```python
from build123d import *

# Parameters (mm, degrees)
EXTRUDE1_DEPTH                                    = 177.8
F_6_32_TAPPED_HOLE1_D                             = 2.7051
F_6_32_TAPPED_HOLE1_DEPTH                         = 9.38784
F_6_32_TAPPED_HOLE1_CBORE_D                       = 3.5052
F_6_32_TAPPED_HOLE1_CBORE_DEPTH                   = 7.0104
F_6_32_TAPPED_HOLE1_TIP                           = 0.81269403
F_6_32_TAPPED_HOLE2_D                             = 2.7051
F_6_32_TAPPED_HOLE2_DEPTH                         = 9.38784
F_6_32_TAPPED_HOLE2_TIP                           = 0.81269403
F_6_32_TAPPED_HOLE3_D                             = 2.7051
F_6_32_TAPPED_HOLE3_DEPTH                         = 9.38784
F_6_32_TAPPED_HOLE3_TIP                           = 0.81269403
CSK_FOR_6_FLAT_HEAD_MACHINE_SCREW_100_D           = 3.7973
CSK_FOR_6_FLAT_HEAD_MACHINE_SCREW_100_DEPTH       = 12.7
CSK_FOR_6_FLAT_HEAD_MACHINE_SCREW_100_CSINK_D     = 7.0866
CSK_FOR_6_FLAT_HEAD_MACHINE_SCREW_100_CSINK_ANGLE = 100
CSK_FOR_6_FLAT_HEAD_MACHINE_SCREW_100_TIP         = 1.140824014


with BuildPart() as part:
    # Sketch1 → Extrude1 (new body)
    with BuildSketch(Plane(origin=(0, 0, 0), x_dir=(1, 0, 0), z_dir=(0, 1, 0))):
        with BuildLine():
            Line((0, -2.54), (0, -101.092))
            ThreePointArc((0, -101.092), (0.743948776, -102.888051224), (2.54, -103.632))
            Line((2.54, -103.632), (50.8, -103.632))
            Line((50.8, -103.632), (50.8, -100.632))
            Line((50.8, -100.632), (5.54, -100.632))
            ThreePointArc((5.54, -100.632), (3.743948776, -99.888051224), (3, -98.092))
            Line((3, -98.092), (3, -5.54))
            ThreePointArc((3, -5.54), (3.743948776, -3.743948776), (5.54, -3))
            Line((5.54, -3), (50.8, -3))
            Line((50.8, -3), (50.8, 0))
            Line((50.8, 0), (2.54, 0))
            ThreePointArc((2.54, 0), (0.743948776, -0.743948776), (0, -2.54))
        make_face()
    extrude(amount=-EXTRUDE1_DEPTH)

    # #6-32 Tapped Hole1
    with Locations(Plane.ZY):
        with Locations((20.066, -12.7), (83.566, -12.7), (83.566, -165.1), (20.066, -165.1)):
            CounterBoreHole(F_6_32_TAPPED_HOLE1_D / 2, F_6_32_TAPPED_HOLE1_CBORE_D / 2, F_6_32_TAPPED_HOLE1_CBORE_DEPTH, depth=F_6_32_TAPPED_HOLE1_DEPTH)
            with Locations((0, 0, -(F_6_32_TAPPED_HOLE1_DEPTH + F_6_32_TAPPED_HOLE1_TIP / 2))):  # 118° drill point
                Cone(0, F_6_32_TAPPED_HOLE1_D / 2, F_6_32_TAPPED_HOLE1_TIP, mode=Mode.SUBTRACT)

    # #6-32 Tapped Hole2
    with Locations(Plane(origin=(0, 0, 0), x_dir=(-1, 0, 0), z_dir=(0, 0, -1))):
        with Locations((-38.1, -12.7), (-38.1, -165.1)):
            Hole(F_6_32_TAPPED_HOLE2_D / 2, depth=F_6_32_TAPPED_HOLE2_DEPTH)
            with Locations((0, 0, -(F_6_32_TAPPED_HOLE2_DEPTH + F_6_32_TAPPED_HOLE2_TIP / 2))):  # 118° drill point
                Cone(0, F_6_32_TAPPED_HOLE2_D / 2, F_6_32_TAPPED_HOLE2_TIP, mode=Mode.SUBTRACT)

    # #6-32 Tapped Hole3
    with Locations(Plane.XY.offset(103.632)):
        with Locations((38.1, -12.7), (38.1, -165.1)):
            Hole(F_6_32_TAPPED_HOLE3_D / 2, depth=F_6_32_TAPPED_HOLE3_DEPTH)
            with Locations((0, 0, -(F_6_32_TAPPED_HOLE3_DEPTH + F_6_32_TAPPED_HOLE3_TIP / 2))):  # 118° drill point
                Cone(0, F_6_32_TAPPED_HOLE3_D / 2, F_6_32_TAPPED_HOLE3_TIP, mode=Mode.SUBTRACT)

    # CSK for #6 Flat Head Machine Screw (100)1
    with Locations(Plane(origin=(0, 0, 0), x_dir=(-1, 0, 0), z_dir=(0, 0, -1))):
        with Locations((-44.45, -171.45), (-44.45, -6.35)):
            CounterSinkHole(CSK_FOR_6_FLAT_HEAD_MACHINE_SCREW_100_D / 2, CSK_FOR_6_FLAT_HEAD_MACHINE_SCREW_100_CSINK_D / 2, depth=CSK_FOR_6_FLAT_HEAD_MACHINE_SCREW_100_DEPTH, counter_sink_angle=CSK_FOR_6_FLAT_HEAD_MACHINE_SCREW_100_CSINK_ANGLE)
            with Locations((0, 0, -(CSK_FOR_6_FLAT_HEAD_MACHINE_SCREW_100_DEPTH + CSK_FOR_6_FLAT_HEAD_MACHINE_SCREW_100_TIP / 2))):  # 118° drill point
                Cone(0, CSK_FOR_6_FLAT_HEAD_MACHINE_SCREW_100_D / 2, CSK_FOR_6_FLAT_HEAD_MACHINE_SCREW_100_TIP, mode=Mode.SUBTRACT)


solid = part.part
```
Model file for the job. Use its own axes, mm. A direction names the side the tool comes from. Coordinates: 2 decimals unless noted, no trailing zeros. Order: outer loops, then holes, each group sorted by start corner. A loop starts at its lowest first (then second) coordinate and runs counter-clockwise, first axis right, second up. Notation, with made-up numbers: (-26.5, 34) - (15.5, 34) arc R19 ccw to (15.5, 69) - close; hole circle Ø7 at (-24, 29). An arc over 180 degrees is marked (long way). Return JSON: item names as keys, results as strings. Group by question number.
1) Probe line 1 (Z direction, x = 29.5, y = -68.5); line 2 (X direction, y = -65, z = 45); line 3 (Y direction, x = 44, z = 2). List the from-to ranges inside material, lowest first. Write a range as from..to.
2) Tool access for faces 4 (the flat face through (3, -88, 52)), 5 (the cylindrical face through (44.038, -173.304, 2.201)), 6 (the cylindrical face through (1.48, -163.92, 82.27)): list every direction of +Z, -Z, +X, -X, +Y, -Y with a clear straight run to the whole face (end or side of a thin tool).
3) Saw through at B-B, the plane y = -6.35. Write the cut outline in (x, z), plus the area to 3 significant figures.
4) Saw through at C-C, the plane x = 44.45. Write the cut outline in (y, z), plus the area to 3 significant figures.
5) Saw through at A-A, the plane x = 9. Write the cut outline in (y, z), plus the area to 3 significant figures.
6) Flat gauge pins, fed straight in: P1, Ø3, axis at x = 38.1, y = -165.1, coming from the -Z side; P2, Ø1.6, axis at x = 38.1, y = -12.7, coming from the +Z side; P3, Ø5.5, axis at y = -165.1, z = 83.566, coming from the +X side. Where does each tip first touch, or does it go through?
7) Saw through at D-D, the plane y = -95.5. Write the cut outline in (x, z), plus the area to 3 significant figures.
8) Mould opens along Y. For faces 1 (the flat face through (2.7, 0, 51.6)), 2 (the cylindrical face through (1.479, -13.371, 21.685)), 3 (the flat face through (0, -88, 51)) say: released by +Y, released by -Y, zero draft, split by the parting line, or undercut.
Values found:
{
 "1": {"line 1": "z = 0..3, 100.63..103.63", "line 2": "x = 0..3", "line 3": "y = -177.8..-173.29, -169.61..-8.19, -4.51..0"},
 "2": {"face 4": "+X, +Y, -Y", "face 5": "-Z", "face 6": "+X, -X"},
 "3": {"outline": "(0, 2.54) arc R2.54 ccw to (2.54, 0) - (40.91, 0) - (42.55, 1.38) - (42.55, 3) - (5.54, 3) arc R2.54 cw to (3, 5.54) - (3, 98.09) arc R2.54 cw to (5.54, 100.63) - (50.8, 100.63) - (50.8, 103.63) - (2.54, 103.63) arc R2.54 ccw to (0, 101.09) - close; (46.35, 1.38) - (47.99, 0) - (50.8, 0) - (50.8, 3) - (46.35, 3) - close", "area": "584 mm²"},
 "4": {"outline": "(-177.8, 0) - (-174.99, 0) - (-173.35, 1.38) - (-173.35, 3) - (-177.8, 3) - close; (-177.8, 100.63) - (0, 100.63) - (0, 103.63) - (-177.8, 103.63) - close; (-169.55, 1.38) - (-167.91, 0) - (-9.89, 0) - (-8.25, 1.38) - (-8.25, 3) - (-169.55, 3) - close; (-4.45, 1.38) - (-2.81, 0) - (0, 0) - (0, 3) - (-4.45, 3) - close", "area": "1,040 mm²"},
 "5": {"outline": "(-177.8, 0) - (0, 0) - (0, 3) - (-177.8, 3) - close; (-177.8, 100.63) - (0, 100.63) - (0, 103.63) - (-177.8, 103.63) - close", "area": "1,070 mm²"},
 "6": {"P1": "stops at z = 0", "P2": "passes through", "P3": "stops at x = 3"},
 "7": {"outline": "(0, 2.54) arc R2.54 ccw to (2.54, 0) - (50.8, 0) - (50.8, 3) - (5.54, 3) arc R2.54 cw to (3, 5.54) - (3, 98.09) arc R2.54 cw to (5.54, 100.63) - (50.8, 100.63) - (50.8, 103.63) - (2.54, 103.63) arc R2.54 ccw to (0, 101.09) - close", "area": "598 mm²"},
 "8": {"face 1": "released by +Y", "face 2": "undercut", "face 3": "zero draft"}
}
